CAD build for the part. Positions are in the model's coordinates, mm. Face numbers are marked on the shaded views. A direction names the side the tool comes from. Round coordinates to 2 decimals unless told otherwise and drop trailing zeros. Order: outer loops, then holes, each group sorted by start corner. A loop starts at its lowest first (then second) coordinate and runs counter-clockwise, first axis right, second up. Notation, with made-up numbers: (31, 26) -> (45, 26) arc R26 ccw to (45, 50) -> close; hole circle Ø3 at (43.25, -16.5). An arc over 180 degrees is marked (long way). Answer as CSV lines item,"result". Start each with the question number.
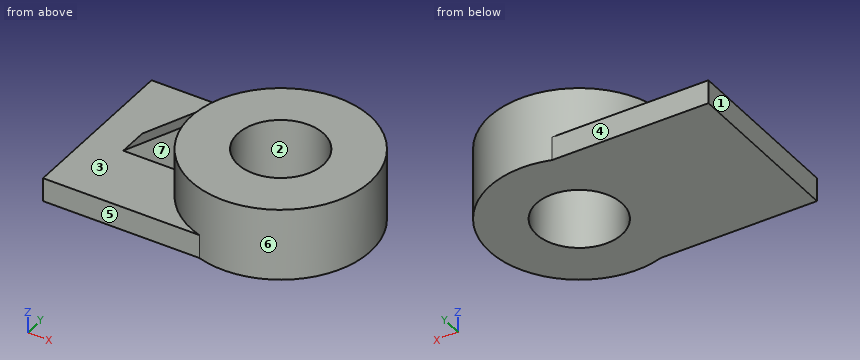
from build123d import *

# Parameters (mm, degrees)
F1_DEPTH = 20.066
F2_R     = 76.246364
F2_R_2   = 36.389637
F3_DEPTH = 61.214
F5_DEPTH = 12.7


with BuildPart() as f1:
    # F0 (on Top) → F1 (new body)
    with BuildSketch(Plane.XY):
        with BuildLine():
            Line((-70.862994, -72.654791), (64.208811, -72.654791))
            ThreePointArc((64.208811, -72.654791), (22.925008, 0), (64.208811, 72.654791))
            Line((64.208811, 72.654791), (-70.862994, 72.654791))
            Line((-70.862994, 72.654791), (-70.862994, -72.654791))
        make_face()
    extrude(amount=F1_DEPTH)

    # F2 (on Top) → F3 (join)
    with BuildSketch(Plane.XY):
        with Locations((85.103318, 0)):
            Circle(F2_R)
        with Locations((85.103318, 0)):
            Circle(F2_R_2, mode=Mode.SUBTRACT)
    extrude(amount=F3_DEPTH)

    # F4 (on Front) → F5 (join, symmetric)
    with BuildSketch(Plane.XZ):
        Polygon((10.999451, 18.561568), (10.082829, 59.809498), (-42.622861, 18.561568), align=None)
    extrude(amount=F5_DEPTH, both=True)


solid = f1.part
Item 1: Pin check, flat tips, straight feed: pin 1 (3 mm diameter, centred on y = -13, z = 18.5, fed in from +X); pin 2 (5 mm diameter, centred on x = 55.5, z = 49.5, fed in from +Y); pin 3 (12 mm diameter, centred on y = -32, z = 49, fed in from +X). Stop position of each tip, or through.
Item 2: Band-saw the part on A-A, the plane x = 109. Give the cut face in (y, z), and give its area (3 significant figures).
Item 3: Band-saw the part on B-B, the plane y = 0. Give the cut face in (x, z).
Item 4: Band-saw the part on C-C, the plane z = 9.5. Give the cut face in (x, y), and give its area (3 significant figures).
Item 5: Probe line 1 (Z direction, x = -19.5, y = 40); line 2 (Y direction, x = 18.5, z = 13); line 3 (Y direction, x = 118, z = 15.5). List the from-to ranges inside material, lowest first.
Item 6: Mould opens along X. For the marked faces 1, 2 and 3 say: released by +X, released by -X, zero draft, split by the parting line, or undercut.
Item 7: Tool access for the marked faces 4, 5, 6 and 7: list every direction of +Z, -Z, +X, -X, +Y, -Y with a clear straight run to the whole face (end or side of a thin tool).
Item 8: Band-saw the part on D-D, the plane y = 41. Give the cut face in (x, z), and give its area (3 significant figures).
Values:
1,pin 1,"x = 160.48"
1,pin 2,"y = 71.27"
1,pin 3,"x = 156.78"
2,outline,"(-72.4, 0) -> (-27.44, 0) -> (-27.44, 61.21) -> (-72.4, 61.21) -> close; (27.44, 0) -> (72.4, 0) -> (72.4, 61.21) -> (27.44, 61.21) -> close"
2,area,"5,500 mm²"
3,outline,"(-70.86, 0) -> (48.71, 0) -> (48.71, 61.21) -> (8.86, 61.21) -> (8.86, 58.85) -> (-40.7, 20.07) -> (-70.86, 20.07) -> close; (121.49, 0) -> (161.35, 0) -> (161.35, 61.21) -> (121.49, 61.21) -> close"
4,outline,"(-70.86, -72.65) -> (61.98, -72.65) arc R76.25 ccw (long way) to (61.98, 72.65) -> (-70.86, 72.65) -> close; hole circle Ø72.78 at (85.1, 0)"
4,area,"27,700 mm²"
5,line 1,"0 to 20.07"
5,line 2,"-72.65 to 72.65"
5,line 3,"-68.78 to -15.56, 15.56 to 68.78"
6,face 1,"released by -X"
6,face 2,"undercut"
6,face 3,"zero draft"
7,face 4,"+Z, -Z, -X, +Y"
7,face 5,"+Z, -Z, -X, -Y"
7,face 6,"+Z"
7,face 7,"+Z, -X, -Y"
8,outline,"(-70.86, 0) -> (149.39, 0) -> (149.39, 61.21) -> (20.82, 61.21) -> (20.82, 20.07) -> (-70.86, 20.07) -> close"
8,area,"9,710 mm²"
